CAD build for the part. Positions are in the model's coordinates, mm. A direction names the side the tool comes from. Give positions to 0.01 mm unless a question says otherwise; leave off trailing zeros. Write each loop counter-clockwise with the first axis right and the second up, starting at its lowest first coordinate (ties: lowest second). Pieces come first, ordered by that corner, then holes. Notation, with made-up numbers: (43.25, 11) -> (66.25, 11) arc R13 ccw to (66.25, 31) -> close; hole circle Ø11 at (43, 88.5). An arc over 180 degrees is marked (long way). Answer as a JSON object with one key per item and string values.
```python
from build123d import *

# Parameters (mm, degrees)
F1_DEPTH = 9
F2_R     = 2.5563686672
F4_DEPTH = 10
F3_R     = 2.6331489766
F5_DEPTH = 10


with BuildPart() as f1:
    # F0 (on Front) → F1 (new body)
    with BuildSketch(Plane.XZ):
        Polygon((-15.2494329959, 47.5306976587), (-53.273987025, 47.5306976587), (-53.273987025, 41.7633611672), (-45.7482971251, 37.4184020777), (-45.7482971251, 28.7284838985), (-53.273987025, 24.383524809), (-53.273987025, 18.6161883175), (-15.2494329959, 18.6161883175), (-15.2494329959, 24.8408854145), (-22.3790369928, 28.9571642013), (-22.3790369928, 37.1897217749), (-15.2494329959, 41.3060005617), align=None)
        Polygon((-45.7482971251, 37.4184020777), (-53.273987025, 41.7633611672), (-53.273987025, 24.383524809), (-45.7482971251, 28.7284838985), align=None)
        Polygon((-53.273987025, 24.383524809), (-53.273987025, 41.7633611672), (-60.7996769249, 37.4184020777), (-60.7996769249, 28.7284838985), align=None)
        Polygon((-8.119828999, 37.1897217749), (-15.2494329959, 41.3060005617), (-15.2494329959, 24.8408854145), (-8.119828999, 28.9571642013), align=None)
        Polygon((-15.2494329959, 24.8408854145), (-15.2494329959, 41.3060005617), (-22.3790369928, 37.1897217749), (-22.3790369928, 28.9571642013), align=None)
    extrude(amount=F1_DEPTH)

    # F2 (on face) → F4 (cut)
    with BuildSketch(Plane.YZ.offset(-8.119828999)):
        with Locations((-4.5300060883, 33.0734429881)):
            Circle(F2_R)
    extrude(amount=-F4_DEPTH, mode=Mode.SUBTRACT)

    # F3 (on face) → F5 (cut)
    with BuildSketch(Plane(origin=(-60.7996769249, 0, 0), x_dir=(0, -1, 0), z_dir=(-1, 0, 0))):
        with Locations((3.9233877324, 33.2661084831)):
            Circle(F3_R)
    extrude(amount=-F5_DEPTH, mode=Mode.SUBTRACT)


solid = f1.part
```
1) Slice it at A-A (y = -0.75). List the corners of the cut face in (x, z), then the cut area to 3 significant figures.
Model answer:
{"outline": "(-60.8, 28.73) -> (-53.27, 24.38) -> (-53.27, 18.62) -> (-15.25, 18.62) -> (-15.25, 24.84) -> (-8.12, 28.96) -> (-8.12, 37.19) -> (-15.25, 41.31) -> (-15.25, 47.53) -> (-53.27, 47.53) -> (-53.27, 41.76) -> (-60.8, 37.42) -> close", "area": "1,290 mm2"}
2) Slice it at D-D (y = -3). List the corners of the cut face in (x, z), then the cut area to 3 significant figures.
Model answer:
{"outline": "(-60.8, 28.73) -> (-53.27, 24.38) -> (-53.27, 18.62) -> (-15.25, 18.62) -> (-15.25, 24.84) -> (-8.12, 28.96) -> (-8.12, 31.03) -> (-18.12, 31.03) -> (-18.12, 35.12) -> (-8.12, 35.12) -> (-8.12, 37.19) -> (-15.25, 41.31) -> (-15.25, 47.53) -> (-53.27, 47.53) -> (-53.27, 41.76) -> (-60.8, 37.42) -> (-60.8, 35.73) -> (-50.8, 35.73) -> (-50.8, 30.8) -> (-60.8, 30.8) -> close", "area": "1,200 mm2"}
3) Wall check: probe 1 along Y at (x, z) = (-16.5, 33); probe 2 along X at (y, z) = (-6.5, 33.5); probe 3 along X at (y, z) = (-6.75, 43.5). Give the ranges that are in metal, low to high.
Model answer:
{"probe 1": "y = -9 to -7.09, -1.97 to 0", "probe 2": "x = -50.8 to -18.12", "probe 3": "x = -53.27 to -15.25"}
4) 3-axis set-ups, long thin cutter, end or side, ignore diameter. For faces 5 (the cylindrical face through (-55.87, -3.353, 30.696)), 6 (the flat face through (-53.274, -4, 22)), 7 (the flat face through (-15.249, -4, 44)): which of +Z, -Z, +X, -X, +Y, -Y reach the whole face in a straight line?
Model answer:
{"face 5": "-X", "face 6": "-Z, -X, +Y, -Y", "face 7": "+Z, +X, +Y, -Y"}
5) Slice it at B-B (z = 34.5). List the corners of the cut face in (x, y), then the cut area to 3 significant figures.
Model answer:
{"outline": "(-60.8, -9) -> (-8.12, -9) -> (-8.12, -6.65) -> (-18.12, -6.65) -> (-18.12, -2.41) -> (-8.12, -2.41) -> (-8.12, 0) -> (-60.8, 0) -> (-60.8, -1.6) -> (-50.8, -1.6) -> (-50.8, -6.25) -> (-60.8, -6.25) -> close", "area": "385 mm2"}
6) Mould opens along Y. For faces 1 (the flat face through (-11.735, -4.437, 26.87)), 2 (the flat face through (-50.8, -4, 33)), 3 (the cylindrical face through (-13.05, -4.86, 35.61)), 4 (the flat face through (-35, 0, 33)) say: released by +Y, released by -Y, zero draft, split by the parting line, or undercut.
Model answer:
{"face 1": "zero draft", "face 2": "undercut", "face 3": "undercut", "face 4": "released by +Y"}
7) Slice it at C-C (x = -52). List the corners of the cut face in (y, z), then the cut area to 3 significant figures.
Model answer:
{"outline": "(-9, 18.62) -> (0, 18.62) -> (0, 47.53) -> (-9, 47.53) -> close; hole circle Ø5.27 at (-3.92, 33.27)", "area": "238 mm2"}
8) Pin check, flat tips, straight feed: pin 1 (1.5 mm diameter, centred on y = -5, z = 33, fed in from +X); pin 2 (3 mm diameter, centred on y = -6, z = 22.5, fed in from -X); pin 3 (3 mm diameter, centred on y = -6.5, z = 22.5, fed in from +X). Stop position of each tip, or through.
Model answer:
{"pin 1": "stops at x = -18.12", "pin 2": "stops at x = -53.27", "pin 3": "stops at x = -15.25"}
